Part model, mm, in its own coordinate system. Coordinates: 2 decimals unless noted, no trailing zeros. Loops run counter-clockwise (first coordinate to the right, second up) from the corner with the lowest first, then second, coordinate; pieces in that order, holes last. Notation, with made-up numbers: (38.5, 5.25) - (45.5, 5.25) arc R18 cw to (45.5, 32.25) - close; hole circle Ø9 at (33.25, 5). An arc over 180 degrees is marked (long way). Answer as CSV lines item,"result".
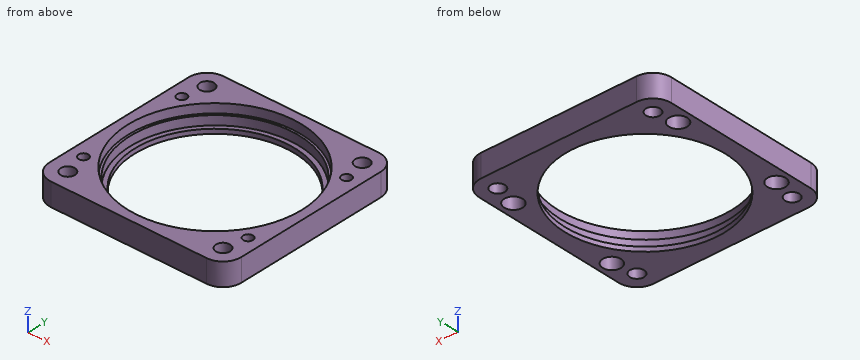
from build123d import *

# Parameters (mm, degrees)
SKETCH_1_W          = 42
SKETCH_1_H          = 42
EXTRUDE_1_DEPTH     = 5
SKETCH_2_R          = 17.5
CUT_EXTRUDE_1_DEPTH = 6
SKETCH_3_R          = 18.5
CUT_EXTRUDE_2_DEPTH = 4
SKETCH_4_R          = 19
CUT_EXTRUDE_3_DEPTH = 2
FILLET_1_R          = 4
SKETCH_5_R          = 1.55
CUT_EXTRUDE_4_DEPTH = 6
SKETCH_7_R          = 1.05
CUT_EXTRUDE_5_DEPTH = 6
SKETCH_8_R          = 2
CUT_EXTRUDE_6_DEPTH = 3


with BuildPart() as part:
    # 草图1 → 凸台-拉伸1 (new body)
    with BuildSketch(Plane.XY):
        Rectangle(SKETCH_1_W, SKETCH_1_H)
    extrude(amount=EXTRUDE_1_DEPTH)

    # 草图2 → 切除-拉伸1 (cut, through all)
    with BuildSketch(Plane.XY.offset(5)):
        Circle(SKETCH_2_R)
    extrude(amount=-CUT_EXTRUDE_1_DEPTH, mode=Mode.SUBTRACT)

    # 草图3 → 切除-拉伸2 (cut)
    with BuildSketch(Plane.XY.offset(5)):
        Circle(SKETCH_3_R)
    extrude(amount=-CUT_EXTRUDE_2_DEPTH, mode=Mode.SUBTRACT)

    # 草图4 → 切除-拉伸3 (cut)
    with BuildSketch(Plane.XY.offset(5)):
        Circle(SKETCH_4_R)
    extrude(amount=-CUT_EXTRUDE_3_DEPTH, mode=Mode.SUBTRACT)

    # 圆角1
    fillet_1_edges = [part.edges().sort_by_distance(p)[0] for p in [
        (21, -21, 2.5),
        (-21, -21, 2.5),
        (-21, 21, 2.5),
        (21, 21, 2.5),
    ]]
    fillet(fillet_1_edges, radius=FILLET_1_R)

    # 草图5 → 切除-拉伸4 (cut, through all)
    with BuildSketch(Plane.XY.offset(5)):
        with Locations((-16.970562748, 16.970562748)):
            Circle(SKETCH_5_R)
        with Locations((16.970562748, 16.970562748)):
            Circle(SKETCH_5_R)
        with Locations((16.970562748, -16.970562748)):
            Circle(SKETCH_5_R)
        with Locations((-16.970562748, -16.970562748)):
            Circle(SKETCH_5_R)
    extrude(amount=-CUT_EXTRUDE_4_DEPTH, mode=Mode.SUBTRACT)

    # 草图7 → 切除-拉伸5 (cut, through all)
    with BuildSketch(Plane(origin=(0, 0, 0), x_dir=(-1, 0, 0), z_dir=(0, 0, -1))):
        with Locations((-18, 12)):
            Circle(SKETCH_7_R)
        with Locations((18, 12)):
            Circle(SKETCH_7_R)
        with Locations((18, -12)):
            Circle(SKETCH_7_R)
        with Locations((-18, -12)):
            Circle(SKETCH_7_R)
    extrude(amount=-CUT_EXTRUDE_5_DEPTH, mode=Mode.SUBTRACT)

    # 草图8 → 切除-拉伸6 (cut)
    with BuildSketch(Plane(origin=(0, 0, 0), x_dir=(-1, 0, 0), z_dir=(0, 0, -1))):
        with Locations((-18, 12)):
            Circle(SKETCH_8_R)
        with Locations((18, 12)):
            Circle(SKETCH_8_R)
        with Locations((18, -12)):
            Circle(SKETCH_8_R)
        with Locations((-18, -12)):
            Circle(SKETCH_8_R)
    extrude(amount=-CUT_EXTRUDE_6_DEPTH, mode=Mode.SUBTRACT)


solid = part.part
Q1. Flat gauge pins, fed straight in: pin 1 (2.5 mm diameter, centred on x = -18, y = -12, fed in from -Z); pin 2 (11 mm diameter, centred on x = -7, y = 2.5, fed in from +Z) (1 decimal). Where does each tip first touch, or does it go through?
Results:
pin 1,"stops at z = 3"
pin 2,"passes through"
Q2. Wall check: L1, parallel to X at y = -0.5, z = 4.3; L2, parallel to X at y = -16, z = 1.05; L3, parallel to Y at x = 0, z = 3.45. Give the ranges that are in metal, low to high.
Results:
L1,"x = -21 to -18.99, 18.99 to 21"
L2,"x = -21 to -18.18, -15.76 to -9.29, 9.29 to 15.76, 18.18 to 21"
L3,"y = -21 to -19, 19 to 21"
Q3. Saw through at C-C (y = 12). Count the separate pieces of the cut face and the enclosed holes in it, then the cut area to 3 significant figures.
Results:
separate pieces,"4"
enclosed holes,"0"
area,"36.9 mm^2"
Q4. Saw through at A-A (x = 0). Give the cut face in (y, z).
Results:
outline,"(-21, 0) - (-17.5, 0) - (-17.5, 1) - (-18.5, 1) - (-18.5, 3) - (-19, 3) - (-19, 5) - (-21, 5) - close; (17.5, 0) - (21, 0) - (21, 5) - (19, 5) - (19, 3) - (18.5, 3) - (18.5, 1) - (17.5, 1) - close"
